The model under review builds one solid part; all positions refer to its coordinate system, in mm. Round coordinates to 2 decimals unless told otherwise and drop trailing zeros. Write each loop counter-clockwise with the first axis right and the second up, starting at its lowest first coordinate (ties: lowest second). Pieces come first, ordered by that corner, then holes. Notation, with made-up numbers: (29.5, 68) - (71.5, 68) arc R24 ccw to (71.5, 104) - close; hole circle Ø8 at (11.5, 51.25). An arc over 180 degrees is marked (long way). Use one line per item in the form item = value.
from build123d import *

# Parameters (mm, degrees)
SKETCH1_W           = 25
SKETCH1_H           = 100
BOSS_EXTRUDE1_DEPTH = 10
SKETCH2_R           = 1
CUT_EXTRUDE1_DEPTH  = 104.561575886


with BuildPart() as part:
    # Sketch1 → Boss-Extrude1 (new body)
    with BuildSketch(Plane.XY):
        with Locations((12.5, 50)):
            Rectangle(SKETCH1_W, SKETCH1_H)
    extrude(amount=BOSS_EXTRUDE1_DEPTH)

    # Sketch2 → Cut-Extrude1 (cut, through all)
    with BuildSketch(Plane.XY.offset(10)):
        with Locations((7.5, 92.5)):
            Circle(SKETCH2_R)
        with Locations((17.5, 47.5)):
            Circle(SKETCH2_R)
        with Locations((7.5, 47.5)):
            Circle(SKETCH2_R)
        with Locations((17.5, 27.5)):
            Circle(SKETCH2_R)
        with Locations((7.5, 27.5)):
            Circle(SKETCH2_R)
        with Locations((17.5, 7.5)):
            Circle(SKETCH2_R)
        with Locations((7.5, 7.5)):
            Circle(SKETCH2_R)
        with Locations(Location((17.5, 92.5, 0), (0, 0, 180))):
            Circle(SKETCH2_R)
    extrude(amount=-CUT_EXTRUDE1_DEPTH, mode=Mode.SUBTRACT)


solid = part.part
(1) Add section A-A on y = 92.5. Write out the cut boundary in (x, z), then the cut area to 3 significant figures.
Geometry results:
outline = (0, 0) - (6.5, 0) - (6.5, 10) - (0, 10) - close; (8.5, 0) - (16.5, 0) - (16.5, 10) - (8.5, 10) - close; (18.5, 0) - (25, 0) - (25, 10) - (18.5, 10) - close
area = 210 mm2
(2) Insertion check: P1, Ø1.2, axis at x = 7.5, y = 92.5, coming from the +Z side. The pin has a flat end and moves straight along its axis. Give the tip position at first contact, or say it passes through.
Geometry results:
P1 = through
(3) To check wall thickness, follow L1, parallel to Y at x = 17.5, z = 5.25; L2, parallel to Y at x = 7, z = 6.25. State the ranges of each line that lie inside material, in increasing order.
Geometry results:
L1 = 0 to 6.5, 8.5 to 26.5, 28.5 to 46.5, 48.5 to 91.5, 93.5 to 100
L2 = 0 to 6.63, 8.37 to 26.63, 28.37 to 46.63, 48.37 to 91.63, 93.37 to 100
(4) The part is to be moulded in two halves that separate along X. For faces 1 (the cylindrical face through (17.04, 93.39, 5.07)), 2 (the flat face through (12, 100, 5)), 3 (the flat face through (25, 49, 5)), say which applies: +X half, -X half, draft (parallel to the pull), parting line (faces both ways), or undercut.
Geometry results:
face_1 = undercut
face_2 = draft
face_3 = +X half
